```python
from build123d import *

# Parameters (mm, degrees)
BOSS_EXTRUDE1_DEPTH = 19.05
CUT_EXTRUDE1_DEPTH  = 12.7
CUT_EXTRUDE2_DEPTH  = 7.62


with BuildPart() as part:
    # Sketch1 → Boss-Extrude1 (new body)
    with BuildSketch(Plane(origin=(0, 0, 0), x_dir=(1, 0, 0), z_dir=(0, 1, 0))):
        Polygon((0, 0), (0, 76.2), (88.9, 76.2), (88.9, 127), (266.7, 127), (266.7, 0), align=None)
    extrude(amount=BOSS_EXTRUDE1_DEPTH)

    # Sketch2 → Cut-Extrude1 (cut)
    with BuildSketch(Plane(origin=(0, 19.05, 0), x_dir=(1, 0, 0), z_dir=(0, 1, 0))):
        Polygon((12.7, 63.5), (101.6, 63.5), (101.6, 114.3), (254, 114.3), (254, 12.7), (12.7, 12.7), align=None)
    extrude(amount=-CUT_EXTRUDE1_DEPTH, mode=Mode.SUBTRACT)

    # Sketch3 → Cut-Extrude2 (cut)
    with BuildSketch(Plane(origin=(0, 19.05, 0), x_dir=(1, 0, 0), z_dir=(0, 1, 0))):
        Polygon((19.05, 76.2), (19.05, 63.5), (101.6, 63.5), (101.6, 107.95), (88.9, 107.95), (88.9, 76.2), align=None)
    extrude(amount=-CUT_EXTRUDE2_DEPTH, mode=Mode.SUBTRACT)


solid = part.part
```
Work out the finished part from the listing and answer in its coordinate system (mm). A direction names the side the tool comes from. Give positions to 0.01 mm unless a question says otherwise; leave off trailing zeros. Order: outer loops, then holes, each group sorted by start corner. A loop starts at its lowest first (then second) coordinate and runs counter-clockwise, first axis right, second up. Notation, with made-up numbers: (53, 11.25) -> (102, 11.25) arc R13 ccw to (102, 27.25) -> close; hole circle Ø3 at (3, -14.5). An arc over 180 degrees is marked (long way). Answer as CSV lines item,"result". Start each with the question number.
(1) Section D-D, the plane z = -82 is taken. Write down the section's boundary in (x, y), plus the area to 3 significant figures.
(2) Section A-A, the plane y = 8.75 is taken. Write down the section's boundary in (x, z).
(3) Consider line 1 along X through (y, z) = (8.25, -85); line 2 along X through (y, z) = (14, -57.5); line 3 along Z through (x, y) = (112, 13.25). Determine where each line is inside the solid, lowest interval first.
(4) This flat-tipped pin is pushed along its axis until it touches: pin 1 Ø9.5 at (x, y) = (46.5, 11.5) entering from -Z. Where does it stop, or does it pass through?
(5) For a pull along Z with two mould halves and no side action, classify faces 4 (the flat face through (177, 13, -114.3)), 5 (the flat face through (135, 9, 0)), 6 (the flat face through (177, 9, -127)), 7 (the flat face through (95, 15, -107.95)) as released by +Z, released by -Z, zero draft, split by the parting line, or undercut.
(6) Section B-B, the plane z = -68.5 is taken. Write down the section's boundary in (x, y).
(7) Section C-C, the plane x = 70 is taken. Write down the section's boundary in (y, z), plus the area to 3 significant figures.
(8) Which of the six approach directions +Z, -Z, +X, -X, +Y, -Y give full straight-line access (tool end or side, diameter ignored) to faces 1 (the flat face through (34, 7, -76.2)), 2 (the flat face through (19.05, 15, -70)), 3 (the flat face through (57, 10, -63.5))?
Entries:
1,outline,"(88.9, 0) -> (266.7, 0) -> (266.7, 19.05) -> (254, 19.05) -> (254, 6.35) -> (101.6, 6.35) -> (101.6, 11.43) -> (88.9, 11.43) -> close"
1,area,"1,350 mm²"
2,outline,"(0, -76.2) -> (88.9, -76.2) -> (88.9, -127) -> (266.7, -127) -> (266.7, 0) -> (0, 0) -> close; hole (12.7, -63.5) -> (101.6, -63.5) -> (101.6, -114.3) -> (254, -114.3) -> (254, -12.7) -> (12.7, -12.7) -> close"
3,line 1,"88.9 to 101.6, 254 to 266.7"
3,line 2,"0 to 12.7, 254 to 266.7"
3,line 3,"-127 to -114.3, -12.7 to 0"
4,pin 1,"z = -76.2"
5,face 4,"undercut"
5,face 5,"released by +Z"
5,face 6,"released by -Z"
5,face 7,"undercut"
6,outline,"(0, 0) -> (266.7, 0) -> (266.7, 19.05) -> (254, 19.05) -> (254, 6.35) -> (101.6, 6.35) -> (101.6, 11.43) -> (19.05, 11.43) -> (19.05, 19.05) -> (0, 19.05) -> close"
7,outline,"(0, -76.2) -> (11.43, -76.2) -> (11.43, -63.5) -> (6.35, -63.5) -> (6.35, -12.7) -> (19.05, -12.7) -> (19.05, 0) -> (0, 0) -> close"
7,area,"710 mm²"
8,face 1,"-Z, -X, +Y, -Y"
8,face 2,"-Z, +Y"
8,face 3,"+Y"
